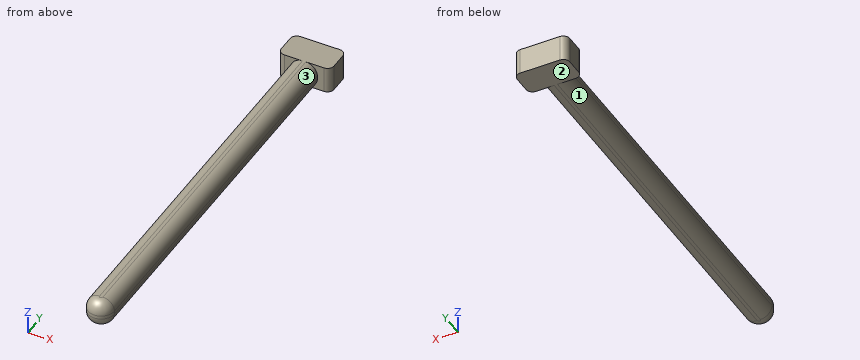
from build123d import *

# Parameters (mm, degrees)
BOSS_EXTRUDE1_DEPTH = 4
FILLET1_R           = 1.75
FILLET2_R           = 1


with BuildPart() as part:
    # Sketch1 → Boss-Extrude1 (new body)
    with BuildSketch(Plane.XY):
        with BuildLine():
            Line((2, -2.25), (-2, -2.25))
            Line((-2, -2.25), (-2, -60))
            ThreePointArc((-2, -60), (0, -62), (2, -60))
            Line((2, -60), (2, -2.25))
        make_face()
        with BuildLine():
            Line((-2, 0), (-2, -2.25))
            Line((-2, -2.25), (2, -2.25))
            Line((2, -2.25), (2, 0))
            ThreePointArc((2, 0), (0, 2), (-2, 0))
        make_face()
        with BuildLine():
            Line((-4, 2.25), (-4, -2.25))
            Line((-4, -2.25), (-2, -2.25))
            Line((-2, -2.25), (-2, 0))
            ThreePointArc((-2, 0), (0, 2), (2, 0))
            Line((2, 0), (2, -2.25))
            Line((2, -2.25), (4, -2.25))
            Line((4, -2.25), (4, 2.25))
            Line((4, 2.25), (-4, 2.25))
        make_face()
    extrude(amount=BOSS_EXTRUDE1_DEPTH)

    # Fillet1
    fillet1_edges = [part.edges().sort_by_distance(p)[0] for p in [
        (2, -31.125, 0),
        (0, -62, 0),
        (-2, -31.125, 0),
        (0, -62, 4),
        (2, -31.125, 4),
        (-2, -31.125, 4),
    ]]
    fillet(fillet1_edges, radius=FILLET1_R)

    # Fillet2
    fillet2_edges = [part.edges().sort_by_distance(p)[0] for p in [
        (-4, -2.25, 2),
        (-4, 2.25, 2),
        (4, 2.25, 2),
        (4, -2.25, 2),
    ]]
    fillet(fillet2_edges, radius=FILLET2_R)


solid = part.part
Geometry check sheet. Reference: the model listing, model coordinates, mm. Face numbers are marked on the shaded views. A direction names the side the tool comes from. Give positions to 0.01 mm unless a question says otherwise; leave off trailing zeros. Loops run counter-clockwise (first coordinate to the right, second up) from the corner with the lowest first, then second, coordinate; pieces in that order, holes last. Notation, with made-up numbers: (-36, 22) -> (-8, 22) arc R20 cw to (-8, 36) -> close; hole circle Ø9 at (69.25, 55). An arc over 180 degrees is marked (long way). Answer in a Markdown table with one row per item. Add a question column.
1) Set-up check for the marked faces 1, 2 and 3: record each of +Z, -Z, +X, -X, +Y, -Y from which the full face is reachable in a straight line by a thin tool's end or side.
2) Cross-section at A-A on y = -49. Record the boundary of the cut face in (x, z).
3) Gauge pin test, flat ends, axial feed: P1, Ø2, axis at y = -42.5, z = 2.5, coming from the +X side; P2, Ø1.5, axis at y = -7, z = 0.5, coming from the -X side; P3, Ø0.8, axis at x = -2.5, z = 2.5, coming from the -Y side. Record the tip position at first contact, or that the pin passes through.
4) Material ranges on probe 1 along X at (y, z) = (-14.5, 2.35); probe 2 along Y at (x, z) = (2.75, 3.75); probe 3 along X at (y, z) = (-22.5, 3.55), recorded low to high. Write a range as from..to.
Outcome:
| question | item | result |
|---|---|---|
| 1 | face 1 | -Z, -X, -Y |
| 1 | face 2 | -Z, +X, -X, +Y, -Y |
| 1 | face 3 | +Z, +X, -Y |
| 2 | outline | (-2, 1.75) arc R1.75 ccw to (-0.25, 0) -> (0.25, 0) arc R1.75 ccw to (2, 1.75) -> (2, 2.25) arc R1.75 ccw to (0.25, 4) -> (-0.25, 4) arc R1.75 ccw to (-2, 2.25) -> close |
| 3 | P1 | stops at x = 2 |
| 3 | P2 | stops at x = -1.93 |
| 3 | P3 | stops at y = -2.25 |
| 4 | probe 1 | x = -2..2 |
| 4 | probe 2 | y = -2.25..2.25 |
| 4 | probe 3 | x = -1.42..1.42 |
